For this review, take the finished solid that the model builds, in its own axes (mm). A direction names the side the tool comes from. Round coordinates to 2 decimals unless told otherwise and drop trailing zeros. Write each loop counter-clockwise with the first axis right and the second up, starting at its lowest first coordinate (ties: lowest second). Pieces come first, ordered by that corner, then holes. Notation, with made-up numbers: M 38.25,-0.5 L 95.25,-0.5 A18 ccw 95.25,29.5 Z; hole C 63.5,54 d8. An arc over 180 degrees is marked long. Use one line per item in the form item = value. Start each with the question number.
Item 1: Draft analysis for pull direction Z (two halves, no side actions). For faces 4 (the flat face through (-15, 0, -19.999)), 5 (the flat face through (3, 5, 0)), 6 (the flat face through (-15, 0, 20.001)), 7 (the flat face through (7.398, 0.07, -15.353)), state which applies: released by +Z, released by -Z, zero draft, split by the parting line, or undercut.
Item 2: For P1, Ø3, axis at y = 0.5, z = 15, coming from the +X side; P2, Ø2, axis at y = 1.5, z = 10, coming from the +X side, all flat-tipped, find the tip position at first contact; note any pin that passes through.
Item 3: Add section C-C (z = 17). State the section outline as (x, y) points, and give its area (3 significant figures).
Item 4: Add section A-A (y = -2.75). Count the separate pieces of the cut face and the enclosed holes in it, and give its area (3 significant figures).
Item 5: For line 1 (Z direction, x = -6, y = -2.5); line 2 (Y direction, x = -11, z = 15.5); line 3 (Z direction, x = -2, y = -1), list the stretches that pass through material, from the lowest coordinate up. Write a range as [from, to].
Item 6: Add section B-B (x = -6.5). State the section outline as (y, z) points, and give its area (3 significant figures).
Item 7: Add section D-D (z = 10). State the section outline as (x, y) points.
Item 8: For faces 1 (the flat face through (-12.67, 0, -12)), 2 (the flat face through (-12.67, 0, 13)), 3 (the flat face through (2, 0, -3.202)), list the 3-axis set-ups (+Z, -Z, +X, -X, +Y, -Y) from which the entire face can be reached by the end or side of a thin tool; tool diameter is ignored.
from build123d import *

# Parameters (mm, degrees)
SALIENTE_EXTRUIR1_DEPTH   = 5
SALIENTE_EXTRUIR1_2_DEPTH = 5
CROQUIS1_W                = 4.860345515
CROQUIS1_H                = 40
SALIENTE_EXTRUIR1_3_DEPTH = 5
SALIENTE_EXTRUIR2_DEPTH   = 2
REDONDEO1_R               = 0.5
REDONDEO2_R               = 0.5
REDONDEO3_R               = 0.5
CROQUIS5_W                = 30.200510783
CROQUIS5_H                = 2
SALIENTE_EXTRUIR3_DEPTH   = 5
REDONDEO4_R               = 0.5
CROQUIS6_W                = 0.06
CROQUIS6_H                = 40
CORTAR_EXTRUIR4_DEPTH     = 17


with BuildPart() as part:
    # Croquis1 → Saliente-Extruir1 (new, symmetric)
    with BuildSketch(Plane(origin=(0, 0, 0), x_dir=(1, 0, 0), z_dir=(0, 1, 0))):
        Polygon((17.530428149, 19.999144472), (-2.49913463, 19.999144472), (-2.53039772, 19.968072403), (-2.53039772, 14.718192691), (17.530428149, 16.000273752), align=None)
    extrude(amount=SALIENTE_EXTRUIR1_DEPTH, both=True)



with BuildPart() as body_2:
    # Croquis1 → Saliente-Extruir1 2 (new, symmetric)
    with BuildSketch(Plane(origin=(0, 0, 0), x_dir=(1, 0, 0), z_dir=(0, 1, 0))):
        Polygon((17.530428149, -20.000855528), (-2.49913463, -20.000855528), (-2.530548466, -19.969634553), (-2.530548466, -14.710829577), (17.530428149, -15.997364244), align=None)
    extrude(amount=SALIENTE_EXTRUIR1_2_DEPTH, both=True)


with BuildPart() as body_3:
    # Croquis1 → Saliente-Extruir1 3 (new, symmetric)
    with BuildSketch(Plane(origin=(0, 0, 0), x_dir=(1, 0, 0), z_dir=(0, 1, 0))):
        with Locations((-15.100255392, -0.000855528)):
            Rectangle(CROQUIS1_W, CROQUIS1_H)
    extrude(amount=SALIENTE_EXTRUIR1_3_DEPTH, both=True)


with BuildPart() as part_1:
    add(part.part)

    add(body_2.part)  # Saliente-Extruir2 merges body 2

    add(body_3.part)  # Saliente-Extruir2 merges body 3
    # Croquis3 → Saliente-Extruir2 (add)
    with BuildSketch(Plane(origin=(0, 5, 0), x_dir=(1, 0, 0), z_dir=(0, 1, 0))):
        with BuildLine():
            Line((-17.530428149, 19.999144472), (-12.670082634, 19.999144472))
            ThreePointArc((-12.670082634, 19.999144472), (-7.615776211, 14.91376598), (-2.53039772, 19.968072403))
            Line((-2.53039772, 19.968072403), (17.530428149, 19.999144472))
            Line((17.530428149, 19.999144472), (17.530428149, -20.000855528))
            Line((17.530428149, -20.000855528), (-2.530548466, -19.969634553))
            ThreePointArc((-2.530548466, -19.969634553), (-7.615926037, -14.915477956), (-12.670082634, -20.000855528))
            Line((-12.670082634, -20.000855528), (-17.530428149, -20.000855528))
            Line((-17.530428149, -20.000855528), (-17.530428149, 19.999144472))
        make_face()
    saliente_extruir2 = extrude(amount=SALIENTE_EXTRUIR2_DEPTH)

    # Simetría1: Saliente-Extruir2 across plane
    add(saliente_extruir2.mirror(Plane.ZX))

    # Redondeo1
    redondeo1_edges = [part_1.edges().sort_by_distance(p)[0] for p in [
        (-2.530548466, 0, 14.710829577),
    ]]
    fillet(redondeo1_edges, radius=REDONDEO1_R)

    # Redondeo2
    redondeo2_edges = [part_1.edges().sort_by_distance(p)[0] for p in [
        (-2.53039772, 0, -14.718192691),
    ]]
    fillet(redondeo2_edges, radius=REDONDEO2_R)

    # Redondeo3
    redondeo3_edges = [part_1.edges().sort_by_distance(p)[0] for p in [
        (17.530428149, 0, 15.997364244),
        (17.530428149, 0, -16.000273752),
    ]]
    fillet(redondeo3_edges, radius=REDONDEO3_R)

    # Croquis5 → Saliente-Extruir3 (add, symmetric)
    with BuildSketch(Plane(origin=(0, 0, 0), x_dir=(1, 0, 0), z_dir=(0, 1, 0))):
        with Locations((2.430172758, -4.198493404)):
            Rectangle(CROQUIS5_W, CROQUIS5_H)
        with Locations((2.430172758, 4.201506596)):
            Rectangle(CROQUIS5_W, CROQUIS5_H)
    extrude(amount=SALIENTE_EXTRUIR3_DEPTH, both=True)

    # Redondeo4
    redondeo4_edges = [part_1.edges().sort_by_distance(p)[0] for p in [
        (17.530428149, 0, -3.201506596),
        (17.530428149, 0, -5.201506596),
        (17.530428149, 0, 5.198493404),
        (17.530428149, 0, 3.198493404),
    ]]
    fillet(redondeo4_edges, radius=REDONDEO4_R)

    # Croquis6 → Cortar-Extruir4 (cut)
    with BuildSketch(Plane(origin=(0, 7, 0), x_dir=(1, 0, 0), z_dir=(0, 1, 0))):
        with Locations((-17.500428149, -0.000855528)):
            Rectangle(CROQUIS6_W, CROQUIS6_H)
    extrude(amount=-CORTAR_EXTRUIR4_DEPTH, mode=Mode.SUBTRACT)


solid = part_1.part
Calculated:
q1.face_4 = released by -Z
q1.face_5 = undercut
q1.face_6 = released by +Z
q1.face_7 = undercut
q2.P1 = 17.53
q2.P2 = -12.67
q3.outline = M -17.47,-7 L -11.7,-7 L -11.7,-5 L -12.67,-5 L -12.67,5 L -11.7,5 L -11.7,7 L -17.47,7 Z; M -3.5,-7 L 17.53,-7 L 17.53,7 L -3.5,7 L -3.5,5 L -2.53,5 L -2.53,-5 L -3.5,-5 Z
q3.area = 356 mm^2
q4.separate_pieces = 3
q4.enclosed_holes = 0
q4.area = 499 mm^2
q5.line_1 = [-5.2, -3.2], [3.2, 5.2]
q5.line_2 = [-7, -5], [5, 7]
q5.line_3 = [-20, -14.75], [-5.2, -3.2], [3.2, 5.2], [14.74, 20]
q6.outline = M -7,-15.03 L -5,-15.03 L -5,-5.2 L 5,-5.2 L 5,-15.03 L 7,-15.03 L 7,15.04 L 5,15.04 L 5,5.2 L -5,5.2 L -5,15.04 L -7,15.04 Z; hole M -5,-3.2 L 5,-3.2 L 5,3.2 L -5,3.2 Z
q6.area = 160 mm^2
q7.outline = M -17.47,-7 L 17.53,-7 L 17.53,-5 L -12.67,-5 L -12.67,5 L 17.53,5 L 17.53,7 L -17.47,7 Z
q8.face_1 = -Z
q8.face_2 = +Z
q8.face_3 = +X
